Check sheet for the drawn part. Datum: minimum x, y, z corner. Units: mm. A direction names the side the tool comes from. Give positions to 0.01 mm unless a question says otherwise; leave off trailing zeros. Write each loop counter-clockwise with the first axis right and the second up, starting at its lowest first coordinate (ties: lowest second). Pieces come first, ordered by that corner, then holes. Notation, with made-up numbers: M -31,30.5 L 20,30.5 A28 cw 20,64.5 Z; hole C 47,38.5 d6. An arc over 180 degrees is marked long. Write item = value, one per line. Start each with the question number.
1) Set-up check for the marked faces 1, 2, 3 and 4: record each of +Z, -Z, +X, -X, +Y, -Y from which the full face is reachable in a straight line by a thin tool's end or side.
2) Sectioned sample at B-B, the plane y = 12. Record the cut outline in (x, z), then the cut area to 3 significant figures.
3) Gauge pin test, flat ends, axial feed: pin 1 (3 mm diameter, centred on x = 10, z = 3, fed in from +Y); pin 2 (1.5 mm diameter, centred on y = 17.5, z = 3.5, fed in from -X); pin 3 (2.5 mm diameter, centred on y = 16, z = 4, fed in from +X); pin 4 (5 mm diameter, centred on x = 12, y = 12, fed in from +Z). Record the tip position at first contact, or that the pin passes through.
4) Sectioned sample at A-A, the plane x = 12. Record the cut outline in (y, z), then the cut area to 3 significant figures.
5) Scan lines: L1, parallel to Y at x = 12, z = 4.45 (3 decimals); L2, parallel to Y at x = 12, z = 3.5; L3, parallel to X at y = 12, z = 4.2. Record each from-to range of solid material in increasing order.
6) Sectioned sample at D-D, the plane y = 6.25. Record the cut outline in (x, z), then the cut area to 3 significant figures.
7) Sectioned sample at C-C, the plane z = 4.5. Record the cut outline in (x, y), then the cut area to 3 significant figures.
8) Draft check along Y on the marked faces 5, 6 and 7. Enter one of: pulls with the +Y half, pulls with the -Y half, needs draft (parallel to the pull), parting line crosses it, or undercut.
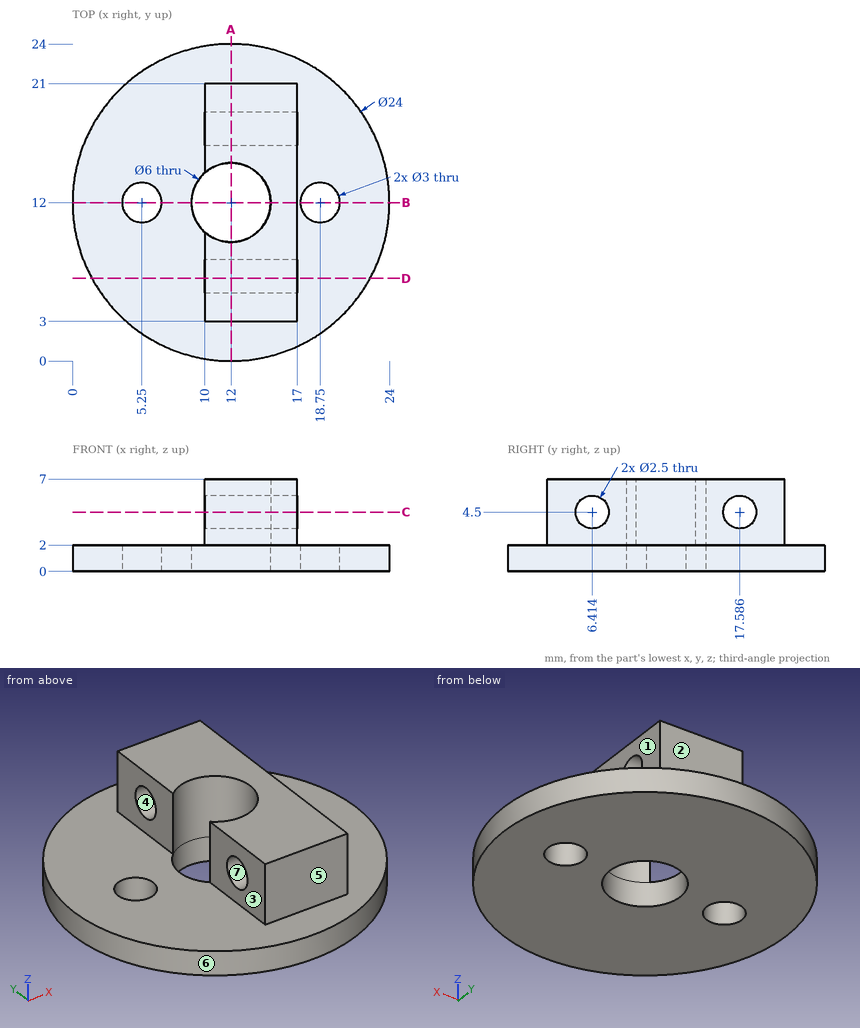
Data:
q1.face_1 = +Z, +X, +Y, -Y
q1.face_2 = +Z, +X, -X, +Y
q1.face_3 = +Z, -X, +Y, -Y
q1.face_4 = +X, -X
q2.outline = M 0,0 L 3.75,0 L 3.75,2 L 0,2 Z; M 6.75,0 L 9,0 L 9,2 L 6.75,2 Z; M 15,0 L 17.25,0 L 17.25,2 L 17,2 L 17,7 L 15,7 Z; M 20.25,0 L 24,0 L 24,2 L 20.25,2 Z
q2.area = 34.0 mm2
q3.pin_1 = 23.97
q3.pin_2 = 10
q3.pin_3 = 17
q3.pin_4 = through
q4.outline = M 0,0 L 9,0 L 9,7 L 3,7 L 3,2 L 0,2 Z; M 15,0 L 24,0 L 24,2 L 21,2 L 21,7 L 15,7 Z; hole C 6.41,4.5 d2.5; hole C 17.59,4.5 d2.5
q4.area = 86.2 mm2
q5.L1 = 3 to 5.165, 7.663 to 9, 15 to 16.337, 18.835 to 21
q5.L2 = 3 to 5.66, 7.16 to 9, 15 to 16.84, 18.34 to 21
q5.L3 = 15 to 17
q6.outline = M 1.47,0 L 22.53,0 L 22.53,2 L 17,2 L 17,3.26 L 10,3.26 L 10,2 L 1.47,2 Z; M 10,5.74 L 17,5.74 L 17,7 L 10,7 Z
q6.area = 59.8 mm2
q7.outline = M 10,3 L 17,3 L 17,5.16 L 10,5.16 Z; M 10,7.66 L 17,7.66 L 17,16.34 L 10,16.34 L 10,14.24 A3 cw long 10,9.76 Z; M 10,18.84 L 17,18.84 L 17,21 L 10,21 Z
q7.area = 65.8 mm2
q8.face_5 = pulls with the -Y half
q8.face_6 = parting line crosses it
q8.face_7 = undercut
